Source: CAD feature listing. Evaluate the final solid. Frame: model axes, mm. A direction names the side the tool comes from. Give positions to 0.01 mm unless a question says otherwise; leave off trailing zeros. Write each loop counter-clockwise with the first axis right and the second up, starting at its lowest first coordinate (ties: lowest second). Pieces come first, ordered by that corner, then holes. Notation, with made-up numbers: M 77.5,-16 L 128.5,-16 A23 cw 128.5,6 Z; hole C 13.25,83.25 d9. An arc over 180 degrees is marked long. Use CSV: the item, a comma, the result in double quotes. Start each with the question number.
from build123d import *

# Parameters (mm, degrees)
SKETCH1_R      = 1.75
SKETCH1_W      = 10.5
SKETCH1_H      = 5
EXTRUDE1_DEPTH = 4.6


with BuildPart() as part:
    # Sketch1 → Extrude1 (new body)
    with BuildSketch(Plane(origin=(0, 0, 0), x_dir=(0, 0, -1), z_dir=(1, 0, 0))):
        with BuildLine():
            Line((20.003411378, 4.993919491), (150.003411378, 4.993919491))
            ThreePointArc((150.003411378, 4.993919491), (160.610013096, 9.387317773), (165.003411378, 19.993919491))
            Line((165.003411378, 19.993919491), (124.610032516, 157.806623844))
            ThreePointArc((124.610032516, 157.806623844), (121.008451259, 162.997888617), (115.013747077, 164.993919491))
            Line((115.013747077, 164.993919491), (90.253411378, 164.993919491))
            Line((90.253411378, 164.993919491), (89.253411378, 163.993919491))
            Line((89.253411378, 163.993919491), (89.253411378, 154.993919491))
            ThreePointArc((89.253411378, 154.993919491), (85.003411378, 150.743919491), (80.753411378, 154.993919491))
            Line((80.753411378, 154.993919491), (80.753411378, 163.993919491))
            Line((80.753411378, 163.993919491), (79.753411378, 164.993919491))
            Line((79.753411378, 164.993919491), (54.993075679, 164.993919491))
            ThreePointArc((54.993075679, 164.993919491), (48.998371496, 162.997888617), (45.39679024, 157.806623844))
            Line((45.39679024, 157.806623844), (5.003411378, 19.993919491))
            ThreePointArc((5.003411378, 19.993919491), (9.39680966, 9.387317773), (20.003411378, 4.993919491))
        make_face()
        with Locations((45.003411378, 9.993919491)):
            Circle(SKETCH1_R, mode=Mode.SUBTRACT)
        with Locations((125.003411378, 9.993919491)):
            Circle(SKETCH1_R, mode=Mode.SUBTRACT)
        with Locations((32.503411378, 9.993919491)):
            Rectangle(SKETCH1_W, SKETCH1_H, mode=Mode.SUBTRACT)
        with Locations((57.503411378, 9.993919491)):
            Rectangle(SKETCH1_W, SKETCH1_H, mode=Mode.SUBTRACT)
        with Locations((137.503411378, 9.993919491)):
            Rectangle(SKETCH1_W, SKETCH1_H, mode=Mode.SUBTRACT)
        with Locations((112.503411378, 9.993919491)):
            Rectangle(SKETCH1_W, SKETCH1_H, mode=Mode.SUBTRACT)
    extrude(amount=EXTRUDE1_DEPTH)


solid = part.part
Item 1: Pull-direction query (Z, two-part tool) for faces 3 (the cylindrical face through (2.268, 9.505, -9.281)), 4 (the cylindrical face through (2.268, 162.944, -121.08)), 5 (the flat face through (2, 7.494, -112)); classes: released by +Z, released by -Z, zero draft, split by the parting line, or undercut.
Item 2: Contact query for flat-ended pins moving along their axis: pin 1 Ø2.5 at (x, y) = (1.5, 10.5) entering from +Z; pin 2 Ø1.4 at (x, y) = (2, 158.5) entering from +Z; pin 3 Ø1.5 at (x, y) = (0.5, 25.5) entering from -Z. Output: stop coordinate, or through.
Item 3: Section D-D (y = 106). Return the cut outline in (x, z).
Item 4: Material intervals for probe 1 along Y at (x, z) = (2.15, -112); probe 2 along Z at (x, y) = (3, 156); probe 3 along Z at (x, y) = (3.35, 135), sorted ascending.
Item 5: Section C-C (z = -135). Return the cut outline in (x, y).
Item 6: Set-up query: faces 1 (the flat face through (2, 10, -62.753)), 2 (the cylindrical face through (2.268, 150.745, -85.097)). Return all of +Z, -Z, +X, -X, +Y, -Y with unobstructed straight access to the full face (end or side cutting, diameter ignored); none if empty.
Item 7: Section A-A (z = -112). Return the cut outline in (x, y), plus the area to 3 significant figures.
Item 8: Section B-B (x = 3.15). State how many separate pieces and enclosed holes the cut face has, plus the area to 3 significant figures.
Output values:
1,face 3,"released by +Z"
1,face 4,"released by -Z"
1,face 5,"undercut"
2,pin 1,"stops at z = -7.47"
2,pin 2,"stops at z = -45.39"
2,pin 3,"stops at z = -163.61"
3,outline,"M 0,-139.79 L 4.6,-139.79 L 4.6,-30.21 L 0,-30.21 Z"
4,probe 1,"y = 4.99 to 7.49, 12.49 to 164.99"
4,probe 2,"z = -125.14 to -89.25, -80.75 to -44.87"
4,probe 3,"z = -131.29 to -38.71"
5,outline,"M 0,4.99 L 4.6,4.99 L 4.6,7.49 L 0,7.49 Z; M 0,12.49 L 4.6,12.49 L 4.6,122.36 L 0,122.36 Z"
6,face 1,"+X, -X"
6,face 2,"+X, -X, +Y"
7,outline,"M 0,4.99 L 4.6,4.99 L 4.6,7.49 L 0,7.49 Z; M 0,12.49 L 4.6,12.49 L 4.6,164.99 L 0,164.99 Z"
7,area,"713 mm2"
8,separate pieces,"1"
8,enclosed holes,"6"
8,area,"19,000 mm2"
